Work out the finished part from the listing and answer in its coordinate system (mm). A direction names the side the tool comes from. Round coordinates to 2 decimals unless told otherwise and drop trailing zeros. Loops run counter-clockwise (first coordinate to the right, second up) from the corner with the lowest first, then second, coordinate; pieces in that order, holes last.
```python
from build123d import *

# Parameters (mm, degrees)
F1_DEPTH       = 28
F3_D           = 4.4
F3_CBORE_D     = 8.25
F3_CBORE_DEPTH = 4


with BuildPart() as f1:
    # F0 (on Front) → F1 (new body)
    with BuildSketch(Plane.XZ):
        with BuildLine():
            Line((-35, -15), (35, -15))
            Line((35, -15), (35, 9))
            Line((35, 9), (19.3406954373, 9))
            ThreePointArc((19.3406954373, 9), (0, -5.25), (-19.3406954373, 9))
            Line((-19.3406954373, 9), (-35, 9))
            Line((-35, 9), (-35, -15))
        make_face()
    extrude(amount=F1_DEPTH)

    # F3 (through all)
    with Locations(Plane.XY.offset(9)):
        with Locations((-28, -5), (-28, -23), (28, -23), (28, -5)):
            CounterBoreHole(F3_D / 2, F3_CBORE_D / 2, F3_CBORE_DEPTH)


solid = f1.part
```
1. Determine the mould class of faces 3 (the face through (-0.5, 0, -5.5)), 4 (the face through (30, -7, 5)), 5 (the face through (35, -14, -3)) for opening direction Y: +Y half, -Y half, draft (parallel to the pull), parting line (faces both ways), or undercut.
Answer key:
face 3: +Y half
face 4: undercut
face 5: draft
2. Find section A-A (z = 7.75). Write down the section's boundary in (x, y) (3 decimals).
Answer key:
outline: (-35, -28) - (-18.908, -28) - (-18.908, 0) - (-35, 0) - close; (18.908, -28) - (35, -28) - (35, 0) - (18.908, 0) - close; hole circle Ø8.25 at (-28, -23); hole circle Ø8.25 at (-28, -5); hole circle Ø8.25 at (28, -23); hole circle Ø8.25 at (28, -5)
3. Find section C-C (z = -7). Write down the section's boundary in (x, y).
Answer key:
outline: (-35, -28) - (35, -28) - (35, 0) - (-35, 0) - close; hole circle Ø4.4 at (-28, -23); hole circle Ø4.4 at (-28, -5); hole circle Ø4.4 at (28, -23); hole circle Ø4.4 at (28, -5)
4. Find section D-D (y = -23). Write down the section's boundary in (x, z) (3 decimals), then the cut area to 3 significant figures.
Answer key:
outline: (-35, -15) - (-30.2, -15) - (-30.2, 5) - (-32.125, 5) - (-32.125, 9) - (-35, 9) - close; (-25.8, -15) - (25.8, -15) - (25.8, 5) - (23.875, 5) - (23.875, 9) - (19.341, 9) arc R20.25 cw to (-19.341, 9) - (-23.875, 9) - (-23.875, 5) - (-25.8, 5) - close; (30.2, -15) - (35, -15) - (35, 9) - (32.125, 9) - (32.125, 5) - (30.2, 5) - close
area: 1,030 mm2
5. Given pin 1 (5 mm diameter, centred on x = -28, y = -23, fed in from +Z); pin 2 (6 mm diameter, centred on x = 11.5, y = -14, fed in from +Z), each flat-ended and moving along its own axis, determine where each tip first touches the part or whether it passes through.
Answer key:
pin 1: stops at z = 5
pin 2: stops at z = 0.86
6. Find section B-B (x = 28). Write down the section's boundary in (y, z) (3 decimals).
Answer key:
outline: (-28, -15) - (-25.2, -15) - (-25.2, 5) - (-27.125, 5) - (-27.125, 9) - (-28, 9) - close; (-20.8, -15) - (-7.2, -15) - (-7.2, 5) - (-9.125, 5) - (-9.125, 9) - (-18.875, 9) - (-18.875, 5) - (-20.8, 5) - close; (-2.8, -15) - (0, -15) - (0, 9) - (-0.875, 9) - (-0.875, 5) - (-2.8, 5) - close
7. Which of the six approach directions +Z, -Z, +X, -X, +Y, -Y give full straight-line access (tool end or side, diameter ignored) to faces 1 (the face through (24.96, -20.21, 7.03)), 2 (the face through (-35, -14, -3))?
Answer key:
face 1: +Z
face 2: +Z, -Z, -X, +Y, -Y
8. Consider probe 1 along Y at (x, z) = (-28, 6.25) (3 decimals); probe 2 along Y at (x, z) = (28, -7.5); probe 3 along X at (y, z) = (-3, 2). Determine where each line is inside the solid, lowest interval first.
Answer key:
probe 1: y = -28 to -27.125, -18.875 to -9.125, -0.875 to 0
probe 2: y = -28 to -25.2, -20.8 to -7.2, -2.8 to 0
probe 3: x = -35 to -28.92, -27.08 to -15.53, 15.53 to 27.08, 28.92 to 35
